Work out the finished part from the listing and answer in its coordinate system (mm). A direction names the side the tool comes from. Coordinates: 2 decimals unless noted, no trailing zeros. Write each loop counter-clockwise with the first axis right and the second up, starting at its lowest first coordinate (ties: lowest second). Pieces come first, ordered by that corner, then holes. Notation, with made-up numbers: (55, 43.5) - (87, 43.5) arc R18 cw to (87, 52.5) - close; hole circle Ø1 at (37, 30.25). An arc over 180 degrees is marked (long way). Answer as a JSON object with one key per item and string values. Group by question number.
from build123d import *

# Parameters (mm, degrees)
SKETCH_2_W           = 50
SKETCH_2_H           = 40
EXTRUDE_1_DEPTH      = 9
EXTRUDE_3_DEPTH      = 5
SKETCH_6_R           = 7.5
CUT_EXTRUDE_1_DEPTH  = 5
SKETCH_7_R           = 3
CUT_EXTRUDE_2_DEPTH  = 34.256578297
CUT_EXTRUDE_START    = -5
CUT_EXTRUDE_11_DEPTH = 5
SKETCH_16_R          = 3
CUT_EXTRUDE_12_DEPTH = 34.256578297


with BuildPart() as part:
    # 草图2 → 凸台-拉伸1 (new body)
    with BuildSketch(Plane(origin=(0, 0, 0), x_dir=(1, 0, 0), z_dir=(0, 1, 0))):
        Rectangle(SKETCH_2_W, SKETCH_2_H)
    extrude(amount=EXTRUDE_1_DEPTH)

    # 草图3 → 凸台-拉伸3 (add)
    with BuildSketch(Plane(origin=(0, 9, 0), x_dir=(1, 0, 0), z_dir=(0, 1, 0))):
        with BuildLine():
            Line((13.5, -15), (-13.5, -15))
            ThreePointArc((-13.5, -15), (-16.328427125, -13.828427125), (-17.5, -11))
            Line((-17.5, -11), (-17.5, 11))
            ThreePointArc((-17.5, 11), (-16.328427125, 13.828427125), (-13.5, 15))
            Line((-13.5, 15), (13.5, 15))
            ThreePointArc((13.5, 15), (16.328427125, 13.828427125), (17.5, 11))
            Line((17.5, 11), (17.5, -11))
            ThreePointArc((17.5, -11), (16.328427125, -13.828427125), (13.5, -15))
        make_face()
    extrude(amount=EXTRUDE_3_DEPTH)

    # 草图6 → 切除-拉伸1 (cut)
    with BuildSketch(Plane(origin=(0, 14, 0), x_dir=(1, 0, 0), z_dir=(0, 1, 0))):
        with Locations(Location((0, 0, 0), (0, 0, 270))):
            Circle(SKETCH_6_R)
    extrude(amount=-CUT_EXTRUDE_1_DEPTH, mode=Mode.SUBTRACT)

    # 草图7 → 切除-拉伸2 (cut, through all)
    with BuildSketch(Plane(origin=(0, 9, 0), x_dir=(1, 0, 0), z_dir=(0, 1, 0))):
        with Locations(Location((0, 0, 0), (0, 0, 270))):
            Circle(SKETCH_7_R)
    extrude(amount=-CUT_EXTRUDE_2_DEPTH, mode=Mode.SUBTRACT)

    # 草图8 → 切除-拉伸11 (cut)
    with BuildSketch(Plane(origin=(0, 14, 0), x_dir=(1, 0, 0), z_dir=(0, 1, 0)).offset(CUT_EXTRUDE_START)):
        with BuildLine():
            ThreePointArc((-8.687466143, 13.218800785), (-7.246696668, 14.526698395), (-5.359264966, 15))
            Line((-5.359264966, 15), (-13.5, 15))
            ThreePointArc((-13.5, 15), (-16.328427125, 13.828427125), (-17.5, 11))
            Line((-17.5, 11), (-17.5, -11))
            ThreePointArc((-17.5, -11), (-16.328427125, -13.828427125), (-13.5, -15))
            Line((-13.5, -15), (-5.359264966, -15))
            ThreePointArc((-5.359264966, -15), (-7.246696668, -14.526698395), (-8.687466143, -13.218800785))
            Line((-8.687466143, -13.218800785), (-16.020799477, -2.218800785))
            ThreePointArc((-16.020799477, -2.218800785), (-16.692598299, 0), (-16.020799477, 2.218800785))
            Line((-16.020799477, 2.218800785), (-8.687466143, 13.218800785))
        make_face()
        with BuildLine():
            ThreePointArc((5.359264966, 15), (7.246696668, 14.526698395), (8.687466143, 13.218800785))
            Line((8.687466143, 13.218800785), (16.020799477, 2.218800785))
            ThreePointArc((16.020799477, 2.218800785), (16.692598299, 0), (16.020799477, -2.218800785))
            Line((16.020799477, -2.218800785), (8.687466143, -13.218800785))
            ThreePointArc((8.687466143, -13.218800785), (7.246696668, -14.526698395), (5.359264966, -15))
            Line((5.359264966, -15), (13.5, -15))
            ThreePointArc((13.5, -15), (16.328427125, -13.828427125), (17.5, -11))
            Line((17.5, -11), (17.5, 11))
            ThreePointArc((17.5, 11), (16.328427125, 13.828427125), (13.5, 15))
            Line((13.5, 15), (5.359264966, 15))
        make_face()
    extrude(amount=CUT_EXTRUDE_11_DEPTH, mode=Mode.SUBTRACT)

    # 草图16 → 切除-拉伸12 (cut, through all)
    with BuildSketch(Plane(origin=(0, 9, 0), x_dir=(1, 0, 0), z_dir=(0, 1, 0))):
        with Locations(Location((-19, 14, 0), (0, 0, 270))):
            Circle(SKETCH_16_R)
        with Locations(Location((-19, -14, 0), (0, 0, 90))):
            Circle(SKETCH_16_R)
        with Locations(Location((19, -14, 0), (0, 0, 270))):
            Circle(SKETCH_16_R)
        with Locations(Location((19, 14, 0), (0, 0, 90))):
            Circle(SKETCH_16_R)
    extrude(amount=-CUT_EXTRUDE_12_DEPTH, mode=Mode.SUBTRACT)


solid = part.part
Q1. Flat-ended cylindrical pins translate along their axes: pin 1 Ø7 at (x, z) = (19, 14) entering from -Y; pin 2 Ø5.5 at (x, z) = (0, 0) entering from +Y; pin 3 Ø1.5 at (x, y) = (-1, 10.5) entering from -Z; pin 4 Ø7.5 at (x, z) = (2.5, -0.5) entering from +Y. Find the tip coordinate at first contact, or state that the pin passes through.
Q2. Section B-B on y = 4.25 is taken. Determine the outline of the cut face in (x, z).
Q3. For a pull along Z with two mould halves and no side action, classify faces 4 (the face through (-20.8, 4.6, -16.4)), 5 (the face through (-7.22, 11.46, 14.54)), 6 (the face through (0, 0, 4)) as +Z half, -Z half, draft (parallel to the pull), parting line (faces both ways), or undercut.
Q4. Section A-A on x = -19 is taken. Determine the outline of the cut face in (y, z).
Q5. Section D-D on y = 11 is taken. Determine the outline of the cut face in (x, z), plus the area to 3 significant figures.
Q6. Consider L1, parallel to X at y = 2, z = -14; L2, parallel to X at y = 5, z = 16.5; L3, parallel to Y at x = 2, z = -2.5. Determine where each line is inside the solid, lowest interval first. Write a range as from..to.
Q7. A tool of negligible diameter and unlimited length cuts with its end or side. For faces 1 (the face through (12.405, 11.465, 7.642)), 2 (the face through (-17, 9, 0)), 3 (the face through (-7.271, 11.465, -14.514)), from which of +Z, -Z, +X, -X, +Y, -Y can it reach the whole face along a straight path? Write none if from no direction.
Q8. Section C-C on z = 0 is taken. Determine the outline of the cut face in (x, y).
Numbers:
{
 "1": {"pin 1": "stops at y = 0", "pin 2": "passes through", "pin 3": "stops at z = -15", "pin 4": "stops at y = 9"},
 "2": {"outline": "(-25, -20) - (25, -20) - (25, 20) - (-25, 20) - close; hole circle Ø6 at (-19, -14); hole circle Ø6 at (-19, 14); hole circle Ø6 at (0, 0); hole circle Ø6 at (19, -14); hole circle Ø6 at (19, 14)"},
 "3": {"face 4": "undercut", "face 5": "+Z half", "face 6": "draft"},
 "4": {"outline": "(0, -20) - (9, -20) - (9, -17) - (0, -17) - close; (0, -11) - (9, -11) - (9, 11) - (0, 11) - close; (0, 17) - (9, 17) - (9, 20) - (0, 20) - close"},
 "5": {"outline": "(-16.02, -2.22) - (-8.69, -13.22) arc R4 ccw to (-5.36, -15) - (5.36, -15) arc R4 ccw to (8.69, -13.22) - (16.02, -2.22) arc R4 ccw to (16.02, 2.22) - (8.69, 13.22) arc R4 ccw to (5.36, 15) - (-5.36, 15) arc R4 ccw to (-8.69, 13.22) - (-16.02, 2.22) arc R4 ccw to start; hole circle Ø15 at (0, 0)", "area": "568 mm²"},
 "6": {"L1": "x = -25..-22, -16..16, 22..25", "L2": "x = -25..-20.66, -17.34..17.34, 20.66..25", "L3": "y = 0..9"},
 "7": {"face 1": "+Z, +X, +Y", "face 2": "+Y", "face 3": "-Z, -X, +Y"},
 "8": {"outline": "(-25, 0) - (-3, 0) - (-3, 9) - (-7.5, 9) - (-7.5, 14) - (-16.69, 14) - (-16.69, 9) - (-25, 9) - close; (3, 0) - (25, 0) - (25, 9) - (16.69, 9) - (16.69, 14) - (7.5, 14) - (7.5, 9) - (3, 9) - close"}
}
